```python
from build123d import *

# Parameters (mm, degrees)
SKETCH_1_W          = 22.4
SKETCH_1_H          = 12.5
EXTRUDE_1_DEPTH     = 22.8
SKETCH_2_W          = 12.5
SKETCH_2_H          = 3
EXTRUDE_2_DEPTH     = 4.7
SKETCH_3_W          = 12.5
SKETCH_3_H          = 3
EXTRUDE_3_DEPTH     = 4.7
SKETCH_4_R          = 1.5
CUT_EXTRUDE_1_DEPTH = 4.7
SKETCH_5_R          = 6.25
EXTRUDE_5_DEPTH     = 3
SKETCH_6_R          = 2
EXTRUDE_6_DEPTH     = 5.1


with BuildPart() as part:
    # 草图1 → 凸台-拉伸1 (new body)
    with BuildSketch(Plane(origin=(0, 0, 0), x_dir=(1, 0, 0), z_dir=(0, 1, 0))):
        with Locations((11.2, -6.25)):
            Rectangle(SKETCH_1_W, SKETCH_1_H)
    extrude(amount=EXTRUDE_1_DEPTH)

    # 草图2 → 凸台-拉伸2 (add)
    with BuildSketch(Plane(origin=(22.4, 0, 0), x_dir=(0, 0, -1), z_dir=(1, 0, 0))):
        with Locations((-6.25, 17.6)):
            Rectangle(SKETCH_2_W, SKETCH_2_H)
    extrude(amount=EXTRUDE_2_DEPTH)

    # 草图3 → 凸台-拉伸3 (add)
    with BuildSketch(Plane.ZY):
        with Locations((6.25, 17.6)):
            Rectangle(SKETCH_3_W, SKETCH_3_H)
    extrude(amount=EXTRUDE_3_DEPTH)

    # 草图4 → 切除-拉伸1 (cut)
    with BuildSketch(Plane(origin=(0, 19.1, 0), x_dir=(1, 0, 0), z_dir=(0, 1, 0))):
        with Locations((-2.65, -6.25)):
            Circle(SKETCH_4_R)
        with Locations((25.05, -6.25)):
            Circle(SKETCH_4_R)
    extrude(amount=-CUT_EXTRUDE_1_DEPTH, mode=Mode.SUBTRACT)

    # 草图5 → 凸台-拉伸5 (add)
    with BuildSketch(Plane(origin=(0, 22.8, 0), x_dir=(1, 0, 0), z_dir=(0, 1, 0))):
        with Locations((6.25, -6.25)):
            Circle(SKETCH_5_R)
    extrude(amount=EXTRUDE_5_DEPTH)

    # 草图6 → 凸台-拉伸6 (add)
    with BuildSketch(Plane(origin=(0, 25.8, 0), x_dir=(1, 0, 0), z_dir=(0, 1, 0))):
        with Locations((6.225516092, -6.25)):
            Circle(SKETCH_6_R)
    extrude(amount=EXTRUDE_6_DEPTH)


solid = part.part
```
Here's how the part is built. I have some questions about the finished solid (model axes, mm). A direction names the side the tool comes from. Round coordinates to 2 decimals unless told otherwise and drop trailing zeros. Write each loop counter-clockwise with the first axis right and the second up, starting at its lowest first coordinate (ties: lowest second). Pieces come first, ordered by that corner, then holes.
Q1. Which directions (+Z, -Z, +X, -X, +Y, -Y) give clear straight access to the entire face, cutting with the end or side of a thin tool? Please do faces 4 (the flat face through (-1.8, 19.1, 4.8)), 5 (the flat face through (6, 25.8, 9)), 6 (the flat face through (25, 19.1, 8)), 7 (the flat face through (1, 22.8, 1)).
Q2. If we section it at C-C on x = 1: Write out the boundary of the cut face in (y, z).
Q3. Will these pins go through, and if not, where does the flat tip stop? P1, Ø5, axis at x = 2.5, z = 2, coming from the +Y side; P2, Ø4, axis at y = 21.5, z = 9, coming from the -X side; P3, Ø1.8, axis at x = -2.65, z = 6.25, coming from the +Y side; P4, Ø2, axis at y = 5.5, z = 6, coming from the +X side.
Q4. If we mould it in two halves opening along Z, with no side actions, what happens to faces 1 (the flat face through (22.4, 8, 6)), 2 (the flat face through (11, 11, 0)), 3 (the cylindrical face through (-1.22, 17.62, 5.8))? For each: +Z half, -Z half, draft (parallel to the pull), parting line (faces both ways), or undercut.
Q5. If we section it at D-D on y = 13: Write out the boundary of the cut face in (x, z).
Q6. If we section it at B-B on z = 2.25: Write out the boundary of the cut face in (x, y), plus the area to 3 significant figures.
Q7. If we section it at A-A on x = -2.65: Write out the boundary of the cut face in (y, z), plus the area to 3 significant figures.
Q8. Please list where these lines run through material, in increasing order: probe 1 along X at (y, z) = (17.95, 6.25); probe 2 along X at (y, z) = (16.5, 5.5); probe 3 along Z at (x, y) = (-2.65, 16.9).
Answer below:
1. face 4: +Z, -Z, -X, +Y
1. face 5: +Y
1. face 6: +Z, -Z, +X, +Y
1. face 7: -Z, -X, +Y
2. outline: (0, 0) - (22.8, 0) - (22.8, 2.86) - (25.8, 2.86) - (25.8, 9.64) - (22.8, 9.64) - (22.8, 12.5) - (0, 12.5) - close
3. P1: stops at y = 25.8
3. P2: stops at x = 0
3. P3: passes through
3. P4: stops at x = 22.4
4. face 1: draft
4. face 2: -Z half
4. face 3: undercut
5. outline: (0, 0) - (22.4, 0) - (22.4, 12.5) - (0, 12.5) - close
6. outline: (-4.7, 16.1) - (0, 16.1) - (0, 0) - (22.4, 0) - (22.4, 16.1) - (27.1, 16.1) - (27.1, 19.1) - (22.4, 19.1) - (22.4, 22.8) - (11.05, 22.8) - (11.05, 25.8) - (1.45, 25.8) - (1.45, 22.8) - (0, 22.8) - (0, 19.1) - (-4.7, 19.1) - close
6. area: 568 mm2
7. outline: (16.1, 0) - (19.1, 0) - (19.1, 4.75) - (16.1, 4.75) - close; (16.1, 7.75) - (19.1, 7.75) - (19.1, 12.5) - (16.1, 12.5) - close
7. area: 28.5 mm2
8. probe 1: x = -4.7 to -4.15, -1.15 to 23.55, 26.55 to 27.1
8. probe 2: x = -4.7 to -3.95, -1.35 to 23.75, 26.35 to 27.1
8. probe 3: z = 0 to 4.75, 7.75 to 12.5
